from build123d import *

# Parameters (mm, degrees)
F1_DEPTH = 4


with BuildPart() as f1:
    # F0 (on Top) → F1 (new body)
    with BuildSketch(Plane.XY):
        Polygon((1000, 0), (0, 0), (0, -193), (2, -193), (2, -336), (248, -336), (248, -193), (250, -193), (252, -193), (252, -336), (498, -336), (498, -193), (500, -193), (502, -193), (502, -336), (748, -336), (748, -193), (750, -193), (752, -193), (752, -336), (998, -336), (998, -193), (1000, -193), align=None)
    extrude(amount=-F1_DEPTH)


solid = f1.part
Geometry: final body of the model. Coordinates: model frame, mm. Round coordinates to 2 decimals unless told otherwise and drop trailing zeros. Order: outer loops, then holes, each group sorted by start corner. A loop starts at its lowest first (then second) coordinate and runs counter-clockwise, first axis right, second up.
Q1. Pin query (flat end, axial travel): pin 1 (1 mm diameter, centred on y = -239.5, z = -2, fed in from -X); pin 2 (1 mm diameter, centred on x = 332, y = -233.5, fed in from +Z); pin 3 (1.2 mm diameter, centred on x = 749, z = -2, fed in from -Y); pin 4 (2 mm diameter, centred on y = -239.5, z = -2.5, fed in from +X). Return the tip coordinate at first contact, or that it passes through.
Result sheet:
pin 1: stops at x = 2
pin 2: stops at z = 0
pin 3: stops at y = -193
pin 4: stops at x = 998
Q2. Section A-A, the plane y = -216. Output: boundary loops of the cut face in (x, z).
Result sheet:
outline: (2, -4) - (248, -4) - (248, 0) - (2, 0) - close; (252, -4) - (498, -4) - (498, 0) - (252, 0) - close; (502, -4) - (748, -4) - (748, 0) - (502, 0) - close; (752, -4) - (998, -4) - (998, 0) - (752, 0) - close
Q3. Material intervals for probe 1 along X at (y, z) = (-266, -2.6), sorted ascending.
Result sheet:
probe 1: x = 2 to 248, 252 to 498, 502 to 748, 752 to 998
